Work out the finished part from the listing and answer in its coordinate system (mm). A direction names the side the tool comes from. Give positions to 0.01 mm unless a question says otherwise; leave off trailing zeros. Write each loop counter-clockwise with the first axis right and the second up, starting at its lowest first coordinate (ties: lowest second). Pieces come first, ordered by that corner, then holes. Notation, with made-up numbers: (15, 34.25) -> (33, 34.25) arc R23 ccw to (33, 65.25) -> close; hole circle Ø10 at (0.5, 75). An arc over 180 degrees is marked (long way). Use a Markdown table: item, result. Add a question column.
Q1. Section D-D, the plane z = 84.5 is taken. Give the vertices of the cut face in (x, y), plus the area to 3 significant figures.
Q2. For a pull along Z with two mould halves and no side action, classify faces 1 (the face through (23.846, -7.509, 27.115)), 2 (the face through (0, 0, 87)), 3 (the face through (0, 0, 83)) as pulls with the +Z half, pulls with the -Z half, needs draft (parallel to the pull), parting line crosses it, or undercut.
Q3. Section A-A, the plane y = 0 is taken. Give the vertices of the cut face in (x, z).
Q4. Each of these flat-tipped pins is pushed along its axis until it touches: pin 1 Ø6 at (y, z) = (-15, 63.5) entering from +X; pin 2 Ø3 at (x, z) = (-8.5, 26) entering from +Y; pin 3 Ø1.5 at (x, z) = (-14, 19.5) entering from +Y; pin 4 Ø1 at (y, z) = (-6.5, 67) entering from +X. Where does it stop, or does it pass through?
Q5. For faces 4 (the face through (1.846, 3.549, 75.846)), 5 (the face through (0, 0, 0)), determine the directions among +Z, -Z, +X, -X, +Y, -Y from which every point of the face is accessible in a straight line to the end or side of a thin tool.
Q6. Consider line 1 (Z direction, x = 0, y = -1.5); line 2 (Z direction, x = -13, y = -0.5); line 3 (X direction, y = 2, z = 84). Determine where each line is inside the solid, lowest interval first.
Q7. Section C-C, the plane z = 72.5 is taken. Give the vertices of the cut face in (x, y).
Q8. Section B-B, the plane x = 0 is taken. Give the vertices of the cut face in (y, z), plus the area to 3 significant figures.
Autodesk Inventor part; units mm, degrees
ref_plane "Work Plane1" through (0, 0, 55) normal (0, 0, 1) x (1, 0, 0)
ref_plane "Work Plane2" through (0, 0, 10) normal (0, 0, -1) x (-1, 0, 0)
ref_plane "YZ Plane" through (0, 0, 0) normal (1, 0, 0) x (0, 1, 0)
sketch "Sketch2" plane through (0, 0, 0) normal (0, 0, 1) x (1, 0, 0)
  circle A0 centre (0, 0) radius 25
  dimension "d0" = 50
extrude "Extrusion1" add sketch "Sketch2" along normal blind 65
sketch "Sketch3" plane through (0, 0, 65) normal (0, 0, 1) x (1, 0, 0)
  circle A0 centre (0, 0) radius 4
  dimension "d3" = 8
extrude "Extrusion2" add sketch "Sketch3" along normal blind 22
ref_plane "Work Plane1" through (0, 0, 55) normal (0, 0, 1) x (1, 0, 0)
ref_plane "Work Plane2" through (0, 0, 10) normal (0, 0, -1) x (-1, 0, 0)
split_face "Split1"
split_face "Split2"
chamfer "Chamfer1" distance 3 distance2 10 1 edges at (-25, 0, 65) measured on face at (17.7191, -2.3134, 65)
sketch "Sketch4" plane through (0, 0, 0) normal (0, 1, 0) x (-1, 0, 0)
  line L0 (4, 87) -> (-4, 87)
  line L1 (-4, 65) -> (4, 65)
  circle A0 centre (0, 84.5) radius 1.5
  point P0 (0, 0)
  dimension "d11" = 3
  dimension "d12" = 2.5
extrude "Extrusion3" cut sketch "Sketch4" along normal through all both and the other way through all
properties part number "Motor" material "Aluminum 6061"
Result set:
| question | item | result |
|---|---|---|
| 1 | outline | (-1.5, -3.71) -> (-1.5, 3.71) arc R4 ccw to start; (1.5, -3.71) arc R4 ccw to (1.5, 3.71) -> close |
| 1 | area | 26.8 mm2 |
| 2 | face 1 | needs draft |
| 2 | face 2 | pulls with the +Z half |
| 2 | face 3 | undercut |
| 3 | outline | (-25, 0) -> (25, 0) -> (25, 55) -> (22, 65) -> (4, 65) -> (4, 87) -> (-4, 87) -> (-4, 65) -> (-22, 65) -> (-25, 55) -> close; hole circle Ø3 at (0, 84.5) |
| 4 | pin 1 | stops at x = 19.25 |
| 4 | pin 2 | stops at y = 24 |
| 4 | pin 3 | stops at y = 21.2 |
| 4 | pin 4 | passes through |
| 5 | face 4 | +Z |
| 5 | face 5 | -Z, +X, -X, +Y, -Y |
| 6 | line 1 | z = 0 to 83, 86 to 87 |
| 6 | line 2 | z = 0 to 65 |
| 6 | line 3 | x = -3.46 to -1.41, 1.41 to 3.46 |
| 7 | outline | circle Ø8 at (0, 0) |
| 8 | outline | (-25, 0) -> (25, 0) -> (25, 55) -> (22, 65) -> (4, 65) -> (4, 83) -> (-4, 83) -> (-4, 65) -> (-22, 65) -> (-25, 55) -> close; (-4, 86) -> (4, 86) -> (4, 87) -> (-4, 87) -> close |
| 8 | area | 3,370 mm2 |
